Can you work these out from the model? Positions are in its coordinate system, mm. Face numbers are marked on the shaded views. A direction names the side the tool comes from. Coordinates: 2 decimals unless noted, no trailing zeros. Loops run counter-clockwise (first coordinate to the right, second up) from the corner with the lowest first, then second, coordinate; pieces in that order, holes last.
```python
from build123d import *

# Parameters (mm, degrees)
SKETCH1_W           = 15
SKETCH1_H           = 10
SKETCH1_H_2         = 15
SKETCH1_W_2         = 10
BOSS_EXTRUDE1_DEPTH = 16.7
SKETCH2_R           = 6.5
CUT_EXTRUDE1_DEPTH  = 8.3
SKETCH3_R           = 6.5
CUT_EXTRUDE2_DEPTH  = 8.3
SKETCH4_R           = 6.5
CUT_EXTRUDE3_DEPTH  = 14.7
BOSS_EXTRUDE2_START = 32
SKETCH5_R           = 6.5
BOSS_EXTRUDE2_DEPTH = 32
BOSS_EXTRUDE3_START = 32
SKETCH6_R           = 6.5
BOSS_EXTRUDE3_DEPTH = 32
BOSS_EXTRUDE4_DEPTH = 16.7
CHAMFER1_SIZE       = 2
CHAMFER2_SIZE       = 2


with BuildPart() as part:
    # Sketch1 → Boss-Extrude1 (new body)
    with BuildSketch(Plane(origin=(0, 0, 0), x_dir=(1, 0, 0), z_dir=(0, 1, 0))):
        Rectangle(SKETCH1_W, SKETCH1_H)
        with Locations((0, 12.5)):
            Rectangle(SKETCH1_W, SKETCH1_H_2)
        with Locations((12.5, 12.5)):
            Rectangle(SKETCH1_W_2, SKETCH1_H_2)
    extrude(amount=BOSS_EXTRUDE1_DEPTH)

    # Sketch2 → Cut-Extrude1 (cut)
    with BuildSketch(Plane.XY.offset(5)):
        with Locations((0, 8.35)):
            Circle(SKETCH2_R)
    extrude(amount=-CUT_EXTRUDE1_DEPTH, mode=Mode.SUBTRACT)

    # Sketch3 → Cut-Extrude2 (cut)
    with BuildSketch(Plane(origin=(17.5, 0, 0), x_dir=(0, 0, -1), z_dir=(1, 0, 0))):
        with Locations((12.5, 8.35)):
            Circle(SKETCH3_R)
    extrude(amount=-CUT_EXTRUDE2_DEPTH, mode=Mode.SUBTRACT)

    # Sketch4 → Cut-Extrude3 (cut)
    with BuildSketch(Plane.XZ):
        with Locations(Location((0, -12.5, 0), (0, 0, 270))):
            Circle(SKETCH4_R)
    extrude(amount=-CUT_EXTRUDE3_DEPTH, mode=Mode.SUBTRACT)

    # Fillet8
    # the kernel refuses this chamfer: 2 mm, written as the material it adds along each edge
    with BuildSketch(Plane(origin=(7.5, 0, -5), x_dir=(-0.027495876610586494, 0, 0.9996219169112968), z_dir=(0, 1, 0))) as fillet8_piece_1:
        with BuildLine():
            Line((2.05734639, 0), (-0.11309431, 2.054235587))
            Line((-0.11309431, 2.054235587), (-0.153079186, 2.053135752))
            ThreePointArc((-0.153079186, 2.053135752), (-0.068258454, 1.026795659), (-0.039984877, -0.001099835))
            Line((-0.039984877, -0.001099835), (0.001099835, -0.039984877))
            ThreePointArc((0.001099835, -0.039984877), (1.028995329, -0.011711299), (2.058446225, -0.039984877))
            Line((2.058446225, -0.039984877), (2.05734639, 0))
        make_face()
    extrude(amount=16.7)
    # the kernel refuses this chamfer: 2 mm, written as the material it takes off along each edge
    with BuildSketch(Plane(origin=(-6.166666667, 1.333333333, -18.666666667), x_dir=(0.7071067811865471, 0, -0.707106781186548), z_dir=(-0.5773502691896263, -0.5773502691896255, -0.5773502691896254)), Plane(origin=(-6.166666667, 15.366666667, -18.666666667), x_dir=(0.7071067811865471, 0.7071067811865478, 0), z_dir=(-0.5773502691896261, 0.5773502691896256, -0.5773502691896256))) as fillet8_2_piece_1:
        Polygon((-1.414213562, -0.816496581), (1.414213562, -0.816496581), (0, 1.632993162), align=None)
    extrude(amount=2.540341184, mode=Mode.SUBTRACT)
    with BuildSketch(Plane(origin=(-7.5, 0, -25.143365976), x_dir=(-0.027495876610586494, 0.9996219169112968, 0), z_dir=(0, 0, 1)), Plane(origin=(22.643365976, 16.7, -20), x_dir=(0, 0.027495876610585647, 0.9996219169112968), z_dir=(-1, 0, 0)), Plane(origin=(-7.5, 16.7, 10.143365976), x_dir=(-0.027495876610586487, -0.9996219169112968, 0), z_dir=(0, 0, -1)), Plane(origin=(22.643365976, 0, -20), x_dir=(0, 0.9996219169112968, -0.02749587661058563), z_dir=(-1, 0, 0))) as fillet8_2_piece_2:
        with BuildLine():
            Line((2.05734639, 0), (-0.11309431, -2.054235587))
            Line((-0.11309431, -2.054235587), (-0.153079186, -2.053135752))
            ThreePointArc((-0.153079186, -2.053135752), (-0.068258454, -1.026795659), (-0.039984877, 0.001099835))
            Line((-0.039984877, 0.001099835), (0.001099835, 0.039984877))
            ThreePointArc((0.001099835, 0.039984877), (1.028995329, 0.011711299), (2.058446225, 0.039984877))
            Line((2.058446225, 0.039984877), (2.05734639, 0))
        make_face()
    extrude(amount=35.286731952, mode=Mode.SUBTRACT)
    with BuildSketch(Plane(origin=(-7.5, -5.143365976, -20), x_dir=(-0.02749587661058694, 0, 0.9996219169112968), z_dir=(0, 1, 0))) as fillet8_2_piece_3:
        with BuildLine():
            Line((2.05734639, 0), (-0.11309431, 2.054235587))
            Line((-0.11309431, 2.054235587), (-0.153079186, 2.053135752))
            ThreePointArc((-0.153079186, 2.053135752), (-0.068258454, 1.026795659), (-0.039984877, -0.001099835))
            Line((-0.039984877, -0.001099835), (0.001099835, -0.039984877))
            ThreePointArc((0.001099835, -0.039984877), (1.028995329, -0.011711299), (2.058446225, -0.039984877))
            Line((2.058446225, -0.039984877), (2.05734639, 0))
        make_face()
    extrude(amount=26.986731952, mode=Mode.SUBTRACT)

    # Sketch5 → Boss-Extrude2 (add)
    with BuildSketch(Plane.XY.offset(5).offset(BOSS_EXTRUDE2_START)):
        Polygon((-7.5, 14.7), (-7.5, 2), (-5.5, 0), (5.5, 0), (7.5, 0), (7.5, 16.7), (5.5, 16.7), (-5.5, 16.7), align=None)
        with Locations((0, 8.35)):
            Circle(SKETCH5_R, mode=Mode.SUBTRACT)
    extrude(amount=-BOSS_EXTRUDE2_DEPTH)

    # Sketch6 → Boss-Extrude3 (add)
    with BuildSketch(Plane(origin=(17.5, 0, 0), x_dir=(0, 0, -1), z_dir=(1, 0, 0)).offset(BOSS_EXTRUDE3_START)):
        Polygon((7, 0), (18, 0), (20, 2), (20, 14.7), (18, 16.7), (7, 16.7), (5, 16.7), (5, 0), align=None)
        with Locations((12.5, 8.35)):
            Circle(SKETCH6_R, mode=Mode.SUBTRACT)
    extrude(amount=-BOSS_EXTRUDE3_DEPTH)

    # Sketch7 → Boss-Extrude4 (add)
    with BuildSketch(Plane(origin=(0, 16.7, 0), x_dir=(1, 0, 0), z_dir=(0, 1, 0))):
        Polygon((7.5, -37), (7.5, 3), (9.5, 5), (49.5, 5), align=None)
    extrude(amount=-BOSS_EXTRUDE4_DEPTH)

    # Chamfer1
    # the kernel refuses this chamfer: 2 mm, written as the material it takes off along each edge
    with BuildSketch(Plane(origin=(49.5, 16.7, 0.143365976), x_dir=(-0.9996219169112968, 0.027495876610585647, 0), z_dir=(0, 0, -1)), Plane(origin=(-10.643365976, 16.7, 37), x_dir=(0, 0.027495876610585647, -0.9996219169112968), z_dir=(1, 0, 0))) as chamfer1_piece_1:
        Polygon((CHAMFER1_SIZE * 0.999621916911, -CHAMFER1_SIZE * 0.0274958766106), (-CHAMFER1_SIZE * 0.0274958766106, -CHAMFER1_SIZE * 0.999621916911), (0, 0), align=None)
    extrude(amount=23.286731952, mode=Mode.SUBTRACT)
    with BuildSketch(Plane(origin=(53.13690896, 16.7, -8.63690896), x_dir=(-0.7068394360706737, 0.027495876610585664, -0.7068394360706735), z_dir=(-0.7071067811865475, 0, 0.7071067811865476))) as chamfer1_piece_2:
        Polygon((CHAMFER1_SIZE * 0.999621916911, CHAMFER1_SIZE * 0.0274958766106), (-CHAMFER1_SIZE * 0.0274958766106, CHAMFER1_SIZE * 0.999621916911), (0, 0), align=None)
    extrude(amount=69.683701572, mode=Mode.SUBTRACT)

    # Chamfer2
    # the kernel refuses this chamfer: 2 mm, written as the material it takes off along each edge
    with BuildSketch(Plane(origin=(53.023839401, 11.176160599, -3.540377928), x_dir=(-0.5328158002121677, -0.1913765872198606, 0.8243071787315372), z_dir=(-0.6785983445455896, 0.6785983445461322, -0.2810846377147535))) as chamfer2_piece_1:
        Polygon((CHAMFER2_SIZE * 0.999945689414, -CHAMFER2_SIZE * 0.0104220066763), (-CHAMFER2_SIZE * 0.858936955191, -CHAMFER2_SIZE * 0.512081348037), (0, 0), align=None)
    extrude(amount=13.332892535, mode=Mode.SUBTRACT)
    with BuildSketch(Plane(origin=(44.512690686, 19.687309314, -15.012690686), x_dir=(0.4218381251250203, -0.39450595107904946, 0.816344076204527), z_dir=(0.5773502691895054, -0.5773502691899669, -0.577350269189405)), Plane(origin=(-10.487309314, 11.712690686, 39.987309314), x_dir=(0.8163440762039974, -0.3945059510795843, 0.4218381251255447), z_dir=(0.5773502691901542, 0.5773502691895923, -0.5773502691891308))) as chamfer2_piece_2:
        Polygon((CHAMFER2_SIZE * 0.999813220622, CHAMFER2_SIZE * 0.0193267656127), (-CHAMFER2_SIZE * 0.516644080304, CHAMFER2_SIZE * 0.856200265292), (0, 0), align=None)
    extrude(amount=13.812444634, mode=Mode.SUBTRACT)
    with BuildSketch(Plane(origin=(7.5, -5.185340786, 37), x_dir=(-0.9998910622590239, 0, 0.014760203742522883), z_dir=(0, 1, 0))) as chamfer2_piece_3:
        Polygon((CHAMFER2_SIZE * 0.999891062259, -CHAMFER2_SIZE * 0.0147602037425), (-CHAMFER2_SIZE * 0.717466790729, -CHAMFER2_SIZE * 0.696592710413), (0, 0), align=None)
    extrude(amount=25.070681572, mode=Mode.SUBTRACT)
    with BuildSketch(Plane(origin=(5.211950804, 20.223839401, 31.476160599), x_dir=(-0.959630861315162, -0.1913765872199142, 0.20611553040850397), z_dir=(0.2810846377147535, -0.6785983445461322, 0.6785983445455896))) as chamfer2_piece_4:
        Polygon((CHAMFER2_SIZE * 0.999945689414, CHAMFER2_SIZE * 0.0104220066763), (-CHAMFER2_SIZE * 0.858936955191, CHAMFER2_SIZE * 0.512081348037), (0, 0), align=None)
    extrude(amount=13.332892535, mode=Mode.SUBTRACT)
    with BuildSketch(Plane(origin=(49.5, -3.143365976, -20), x_dir=(0.027495876610585647, 0, 0.9996219169112968), z_dir=(0, 1, 0)), Plane(origin=(-7.5, 19.843365976, 37), x_dir=(0.9996219169112968, 0, 0.027495876610585623), z_dir=(0, -1, 0))) as chamfer2_piece_5:
        Polygon((CHAMFER2_SIZE * 0.999621916911, -CHAMFER2_SIZE * 0.0274958766106), (-CHAMFER2_SIZE * 0.0274958766106, -CHAMFER2_SIZE * 0.999621916911), (0, 0), align=None)
    extrude(amount=22.986731952, mode=Mode.SUBTRACT)
    with BuildSketch(Plane(origin=(49.5, 19.885340786, -5), x_dir=(-0.6965927104131439, 0, 0.7174667907292085), z_dir=(0, -1, 0))) as chamfer2_piece_6:
        Polygon((CHAMFER2_SIZE * 0.999891062259, CHAMFER2_SIZE * 0.0147602037425), (-CHAMFER2_SIZE * 0.717466790729, CHAMFER2_SIZE * 0.696592710413), (0, 0), align=None)
    extrude(amount=25.070681572, mode=Mode.SUBTRACT)


solid = part.part
```
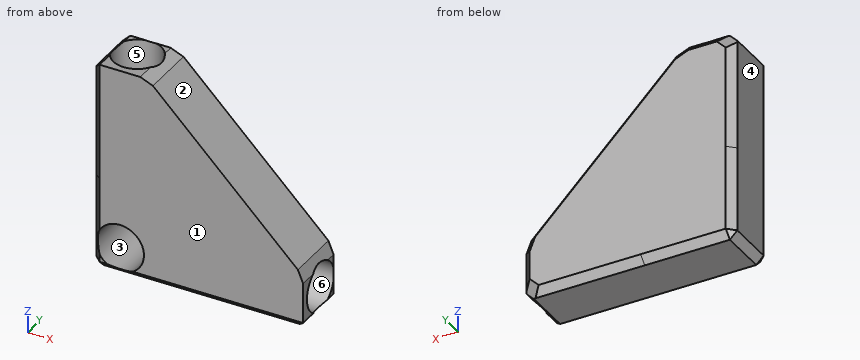
Item 1: Suppose I cut it at B-B, the plane x = 0. Please give me the cut outline in (y, z), plus the area to 3 significant figures.
Results are:
outline: (0, -6) - (14.7, -6) - (14.7, -19) - (1, -19) - (2, -20) - (14.7, -20) - (16.7, -18) - (16.7, 35) - (14.85, 36.85) - (14.85, -3.3) - (1.85, -3.3) - (1.85, 37) - (0, 37) - close
area: 231 mm2
Item 2: We'd pull the mould along X, two halves only. Please class the marked faces 1, 2 and 3: +X half, -X half, draft (parallel to the pull), parting line (faces both ways), or undercut.
Results are:
face 1: draft
face 2: +X half
face 3: undercut
Item 3: I'm going to push flat-ended pins straight in: P1, Ø4, axis at x = -2.5, y = 7.5, coming from the +Z side; P2, Ø6.5, axis at x = -2.5, z = -11, coming from the -Y side; P3, Ø1.5, axis at x = 15.5, y = 9, coming from the +Z side. Where does each tip first touch, or does it pass through?
Results are:
P1: stops at z = -3.3
P2: stops at y = 14.7
P3: stops at z = 29.75
Item 4: On a 3-axis mill with a long thin cutter (end or side, diameter ignored), from which of +Z, -Z, +X, -X, +Y, -Y can I reach the whole of each face in a straight line? I mean the marked faces 4, 5 and 6. Say none if no direction works.
Results are:
face 4: +Z, -Z, -X, +Y, -Y
face 5: +Z
face 6: +X
Item 5: Suppose I cut it at A-A, the plane z = 21.5. Please give me the cut outline in (x, y).
Results are:
outline: (-7.5, 2) - (-5.5, 0) - (23, 0) - (23, 14.7) - (20.17, 16.7) - (-5.5, 16.7) - (-7.5, 14.7) - close; hole circle Ø13 at (0, 8.35)
Item 6: I need wall thicknesses on line 1 along X through (y, z) = (11, -12.5); line 2 along Y through (x, z) = (5.5, 8); line 3 along Z through (x, y) = (0, 4.75). Which ranges of each line are inside material? Lowest first, please.
Results are:
line 1: x = -7.5 to -6.5, 6.5 to 9.2
line 2: y = 0 to 4.89, 11.81 to 16.7
line 3: z = -20 to -19, -6 to -3.3
Item 7: Suppose I cut it at C-C, the plane y = 8.35. Please give me the cut outline in (x, z), plus the area to 3 significant figures.
Results are:
outline: (-7.5, -18) - (-5.5, -20) - (47.5, -20) - (48.5, -19) - (9.2, -19) - (9.2, -6) - (49.09, -6) - (48.09, -3.59) - (8.91, 35.59) - (6.5, 36.59) - (6.5, -3.3) - (-6.5, -3.3) - (-6.5, 36) - (-7.5, 35) - close; hole circle Ø13 at (0, -12.5)
area: 1,180 mm2
Item 8: Suppose I cut it at D-D, the plane x = 39.5. Please give me the cut outline in (y, z).
Results are:
outline: (0, -18) - (2, -20) - (14.7, -20) - (16.7, -18) - (16.7, 2.17) - (14.7, 5) - (0, 5) - close; hole circle Ø13 at (8.35, -12.5)
